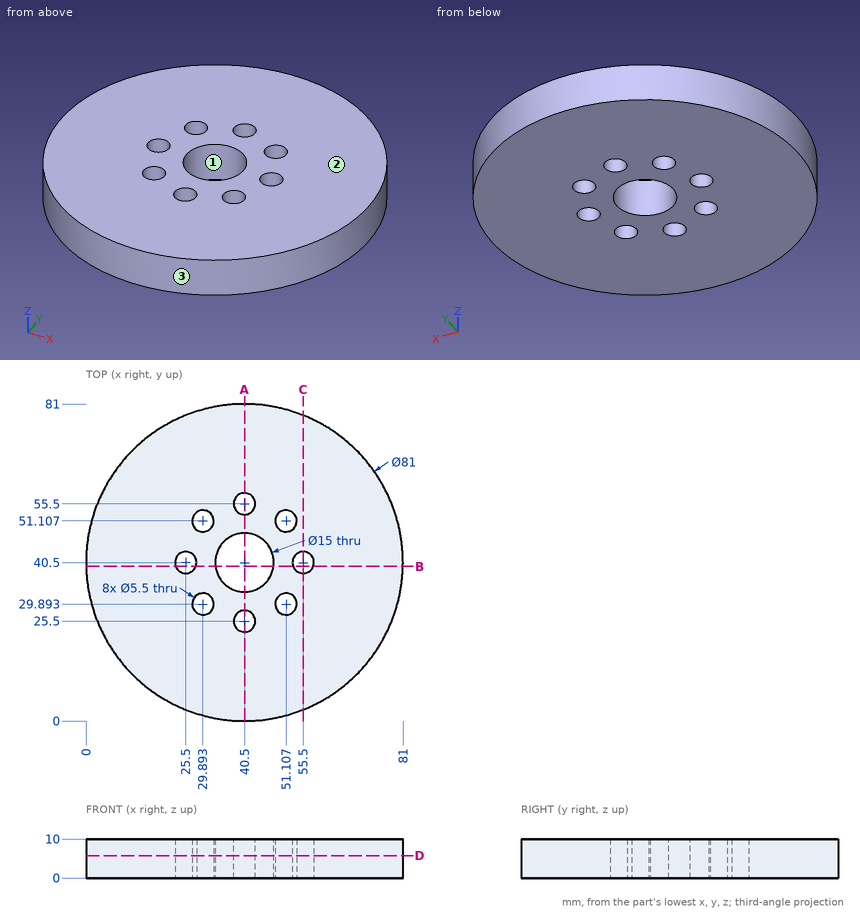
Design review of the part shown in the three views and the two pictorial views. Dimensions are in mm from the part's minimum x, y and z. Round coordinates to 2 decimals unless told otherwise and drop trailing zeros. Write each loop counter-clockwise with the first axis right and the second up, starting at its lowest first coordinate (ties: lowest second). Pieces come first, ordered by that corner, then holes. Notation, with made-up numbers: (26.25, 50.5) - (37.25, 50.5) arc R22 ccw to (37.25, 82.5) - close; hole circle Ø7 at (-32, -12). An arc over 180 degrees is marked (long way). Answer as CSV lines item,"result". Start each with the question number.
(1) Add section B-B, the plane y = 39.5. State the section outline as (x, z) points.
(2) Add section D-D, the plane z = 5.75. State how many separate pieces and enclosed holes the cut face has, plus the area to 3 significant figures.
(3) For pin 1 (3.5 mm diameter, centred on x = 29.89, y = 51.11, fed in from -Z); pin 2 (3 mm diameter, centred on x = 41, z = 5, fed in from +Y); pin 3 (6 mm diameter, centred on y = 14, z = 6.5, fed in from +X) (1 decimal); pin 4 (1.5 mm diameter, centred on y = 71.5, z = 2.5, fed in from +X), all flat-tipped, find the tip position at first contact; note any pin that passes through.
(4) For line 1 (Y direction, x = 40.5, z = 7.75); line 2 (Y direction, x = 28.5, z = 7.5) (1 decimal); line 3 (Y direction, x = 55, z = 2.25) (1 decimal), list the stretches that pass through material, from the lowest coordinate up.
(5) Mouldability with a two-part tool opening along Y and no side actions: class the marked faces 1, 2 and 3 as +Y half, -Y half, draft (parallel to the pull), parting line (faces both ways), or undercut.
(6) Add section A-A, the plane x = 40.5. State the section outline as (y, z) points.
(7) Add section C-C, the plane x = 55.5. State the section outline as (y, z) points.
From the geometry:
1,outline,"(0.01, 0) - (22.94, 0) - (22.94, 10) - (0.01, 10) - close; (28.06, 0) - (33.07, 0) - (33.07, 10) - (28.06, 10) - close; (47.93, 0) - (52.94, 0) - (52.94, 10) - (47.93, 10) - close; (58.06, 0) - (80.99, 0) - (80.99, 10) - (58.06, 10) - close"
2,separate pieces,"1"
2,enclosed holes,"9"
2,area,"4,790 mm²"
3,pin 1,"passes through"
3,pin 2,"stops at y = 81"
3,pin 3,"stops at x = 73.5"
3,pin 4,"stops at x = 67.43"
4,line 1,"y = 0 to 22.75, 28.25 to 33, 48 to 52.75, 58.25 to 81"
4,line 2,"y = 1.8 to 27.5, 32.3 to 48.7, 53.5 to 79.2"
4,line 3,"y = 2.7 to 37.8, 43.2 to 78.3"
5,face 1,"undercut"
5,face 2,"draft"
5,face 3,"parting line"
6,outline,"(0, 0) - (22.75, 0) - (22.75, 10) - (0, 10) - close; (28.25, 0) - (33, 0) - (33, 10) - (28.25, 10) - close; (48, 0) - (52.75, 0) - (52.75, 10) - (48, 10) - close; (58.25, 0) - (81, 0) - (81, 10) - (58.25, 10) - close"
7,outline,"(2.88, 0) - (37.75, 0) - (37.75, 10) - (2.88, 10) - close; (43.25, 0) - (78.12, 0) - (78.12, 10) - (43.25, 10) - close"
